```python
from build123d import *

# Parameters (mm, degrees)
F0_R     = 152.4
F1_DEPTH = 100
F2_R     = 254
F2_R_2   = 152.4
F3_DEPTH = 1000
F4_R     = 152.4
F5_DEPTH = 100


with BuildPart() as f1:
    # F0 (on Top) → F1 (new body)
    with BuildSketch(Plane.XY):
        Circle(F0_R)
    extrude(amount=F1_DEPTH)

    # F2 (on face) → F3 (join)
    with BuildSketch(Plane(origin=(0, 0, 0), x_dir=(1, 0, 0), z_dir=(0, 0, -1))):
        Circle(F2_R)
        Circle(F2_R_2, mode=Mode.SUBTRACT)
        Circle(F2_R_2)
    extrude(amount=F3_DEPTH)

    # F4 (on face) → F5 (join)
    with BuildSketch(Plane(origin=(0, 0, -1000), x_dir=(1, 0, 0), z_dir=(0, 0, -1))):
        Circle(F4_R)
    extrude(amount=F5_DEPTH)


solid = f1.part
```
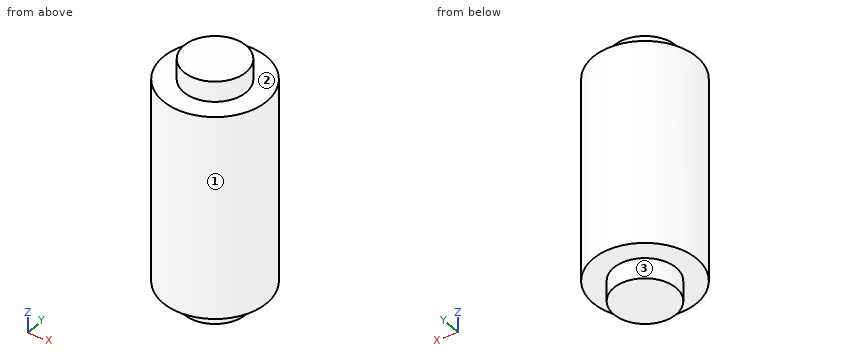
Work out the finished part from the listing and answer in its coordinate system (mm). Face numbers are marked on the shaded views. A direction names the side the tool comes from. Coordinates: 2 decimals unless noted, no trailing zeros. Loops run counter-clockwise (first coordinate to the right, second up) from the corner with the lowest first, then second, coordinate; pieces in that order, holes last. Notation, with made-up numbers: (79.5, -17) -> (124.5, -17) arc R9 cw to (124.5, -1) -> close; hole circle Ø8 at (26, 18.25). An arc over 180 degrees is marked (long way). Answer as CSV lines item,"result".
Q1. The part is cut by section D-D on x = 203. Write down the section's boundary in (y, z), and give its area (3 significant figures).
Findings:
outline,"(-152.67, -1000) -> (152.67, -1000) -> (152.67, 0) -> (-152.67, 0) -> close"
area,"305,000 mm²"
Q2. A tool of negligible diameter and unlimited length cuts with its end or side. For the marked faces 1, 2 and 3, from which of +Z, -Z, +X, -X, +Y, -Y can it reach the whole face along a straight path? Write none if from no direction.
Findings:
face 1,"+Z, -Z"
face 2,"+Z"
face 3,"-Z"
Q3. Each of these flat-tipped pins is pushed along its axis until it touches: pin 1 (10 mm diameter, centred on y = -154.5, z = -752.5, fed in from +X); pin 2 (2 mm diameter, centred on x = -158, y = 86, fed in from -Z); pin 3 (8 mm diameter, centred on x = 90.5, z = -662, fed in from +Y). Where does it stop, or does it pass through?
Findings:
pin 1,"stops at x = 205.34"
pin 2,"stops at z = -1000"
pin 3,"stops at y = 238.82"
Q4. The part is cut by section C-C on z = -336. Write down the section's boundary in (x, y), and give its area (3 significant figures).
Findings:
outline,"circle Ø508 at (0, 0)"
area,"203,000 mm²"
Q5. The part is cut by section A-A on x = 0. Write down the section's boundary in (y, z).
Findings:
outline,"(-254, -1000) -> (-152.4, -1000) -> (-152.4, -1100) -> (152.4, -1100) -> (152.4, -1000) -> (254, -1000) -> (254, 0) -> (152.4, 0) -> (152.4, 100) -> (-152.4, 100) -> (-152.4, 0) -> (-254, 0) -> close"
Q6. Find the intervals of material crossed by probe 1 along Y at (x, z) = (-1.5, -326); probe 2 along Z at (x, y) = (112.5, -207.5); probe 3 along X at (y, z) = (-29, -291.5), in increasing order.
Findings:
probe 1,"y = -254 to 254"
probe 2,"z = -1000 to 0"
probe 3,"x = -252.34 to 252.34"
